Geometry check sheet. Reference: the model listing, model coordinates, mm. A direction names the side the tool comes from. Give positions to 0.01 mm unless a question says otherwise; leave off trailing zeros. Write each loop counter-clockwise with the first axis right and the second up, starting at its lowest first coordinate (ties: lowest second). Pieces come first, ordered by that corner, then holes. Notation, with made-up numbers: (60, 18) - (97, 18) arc R36 cw to (97, 53) - close; hole circle Ø7 at (66, -7.5). An arc over 180 degrees is marked (long way). One line per question, with ' | ' between items. Start each with the question number.
Q1. Section check C-C on y = -13.5. Record the boundary of the cut face in (x, z), and give its area (3 significant figures).
Q2. Thickness scan on L1, parallel to Z at x = 0.6, y = 0 (1 decimal); L2, parallel to Y at x = 1.35, z = -37; L3, parallel to Z at x = 1.4, y = -0.5 (3 decimals). Record the ranges inside material, lowest first. Write a range as [from, to].
Q3. Gauge pin test, flat ends, axial feed: P1, Ø0.5, axis at x = 0.5, y = -18, coming from the -Z side; P2, Ø1.9, axis at y = 12.7, z = 0, coming from the -X side; P3, Ø0.8, axis at x = 1, z = -30.5, coming from the +Y side. Record the tip position at first contact, or that the pin passes through.
Q4. Section check A-A on z = 0. Record the boundary of the cut face in (x, y) (1 decimal), and give its area (3 significant figures).
Q5. Set-up check for faces 4 (the face through (1, 18, -12.7)), 5 (the face through (1, -18, -12.7)), 6 (the face through (1, 0, 12.7)): record each of +Z, -Z, +X, -X, +Y, -Y from which the full face is reachable in a straight line by a thin tool's end or side.
Q6. Section check D-D on z = -21.5. Record the boundary of the cut face in (x, y).
Q7. Section check B-B on y = 0. Record the boundary of the cut face in (x, z) (1 decimal), and give its area (3 significant figures).
Q8. Release check for a two-part mould opening along Z. For faces 1 (the face through (1, -12.7, -30)), 2 (the face through (0.783, -0.344, -39.725)), 3 (the face through (1, 0, -47.625)) record: +Z half, -Z half, draft (parallel to the pull), parting line (faces both ways), or undercut.
Autodesk Inventor part; units mm, degrees
ref_plane "YZ Plane" through (0, 0, 0) normal (1, 0, 0) x (0, 1, 0)
ref_plane "XZ Plane" through (0, 0, 0) normal (0, 1, 0) x (-1, 0, 0)
ref_plane "XY Plane" through (0, 0, 0) normal (0, 0, 1) x (1, 0, 0)
sketch "Sketch1" plane through (0, 0, 0) normal (1, 0, 0) x (0, 1, 0)
  line L0 (0, 0) -> (0, -41.275) construction
  circle A0 centre (0, -22.225) radius 1.5875
  circle A1 centre (0, -41.275) radius 1.5875
  line L1 (22.225, 12.7) -> (22.225, -12.7)
  line L2 (22.225, -12.7) -> (12.7, -12.7)
  line L3 (12.7, -12.7) -> (12.7, -47.625)
  line L4 (12.7, -47.625) -> (-12.7, -47.625)
  line L5 (-22.225, 12.7) -> (22.225, 12.7)
  line L6 (0, -41.275) -> (0, -47.625) construction
  line L7 (12.7, 0) -> (-12.7, 0) construction
  circle A2 centre (12.7, 0) radius 1.5875
  circle A3 centre (-12.7, 0) radius 1.5875
  line L8 (-22.225, 12.7) -> (-22.225, -12.7)
  line L9 (-22.225, -12.7) -> (-12.7, -12.7)
  line L10 (-12.7, -12.7) -> (-12.7, -47.625)
  dimension "d2" = 22.225
  dimension "d3" = 19.05
  dimension "d4" = 25.4
  dimension "d5" = 6.35
  dimension "d9" = 3.175
  dimension "d10" = 25.4
  dimension "d11" = 9.525
  dimension "d12" = 12.7
extrude "Extrusion1" add sketch "Sketch1" along normal blind 1.5875
properties part number "L Plate" material "Aluminum 6061"
Working result:
1) outline: (0, -12.7) - (1.59, -12.7) - (1.59, -1.37) - (0, -1.37) - close; (0, 1.37) - (1.59, 1.37) - (1.59, 12.7) - (0, 12.7) - close | area: 36.0 mm2
2) L1: z = [-47.6, -42.9], [-39.7, -23.8], [-20.6, 12.7] | L2: y = [-12.7, 12.7] | L3: z = [-47.625, -42.782], [-39.768, -23.732], [-20.718, 12.7]
3) P1: stops at z = -12.7 | P2: passes through | P3: stops at y = 12.7
4) outline: (0, -22.2) - (1.6, -22.2) - (1.6, -14.3) - (0, -14.3) - close; (0, -11.1) - (1.6, -11.1) - (1.6, 11.1) - (0, 11.1) - close; (0, 14.3) - (1.6, 14.3) - (1.6, 22.2) - (0, 22.2) - close | area: 60.5 mm2
5) face 4: -Z, +X, -X, +Y | face 5: -Z, +X, -X, -Y | face 6: +Z, +X, -X, +Y, -Y
6) outline: (0, -12.7) - (1.59, -12.7) - (1.59, -1.41) - (0, -1.41) - close; (0, 1.41) - (1.59, 1.41) - (1.59, 12.7) - (0, 12.7) - close
7) outline: (0, -47.6) - (1.6, -47.6) - (1.6, -42.9) - (0, -42.9) - close; (0, -39.7) - (1.6, -39.7) - (1.6, -23.8) - (0, -23.8) - close; (0, -20.6) - (1.6, -20.6) - (1.6, 12.7) - (0, 12.7) - close | area: 85.7 mm2
8) face 1: draft | face 2: undercut | face 3: -Z half
